```python
from build123d import *

# Parameters (mm, degrees)
SKETCH1_R               = 6.477
BOSS_EXTRUDE1_DEPTH     = 2.032
CUT_EXTRUDE1_DEPTH      = 0.64008
SKETCH3_W               = 1.19888
SKETCH3_H               = 8.98144
CUT_EXTRUDE2_DEPTH      = 1.09982
SKETCH4_W               = 7.19836
SKETCH4_H               = 7.00786
CUT_EXTRUDE3_DEPTH      = 0.8001
BOSS_EXTRUDE2_DEPTH     = 1.27
SKETCH6_W               = 2.286
SKETCH6_H               = 1.99898
BOSS_EXTRUDE3_DEPTH     = 2.54
SKETCH7_R               = 3.3734375
BOSS_EXTRUDE4_DEPTH     = 2.032
SKETCH8_W               = 2.54
SKETCH8_H               = 0.79375
CUT_EXTRUDE4_DEPTH      = 1
CUT_EXTRUDE4_DEPTH_BACK = 29.6004
CHAMFER1_SIZE           = 1.143
CHAMFER2_SIZE           = 1.143


with BuildPart() as part:
    # Sketch1 → Boss-Extrude1 (new body)
    with BuildSketch(Plane(origin=(0, 0, 0), x_dir=(1, 0, 0), z_dir=(0, 1, 0))):
        with BuildLine():
            Line((-14.3002, 5.9944), (-14.3002, -24.3332))
            Line((-14.3002, -24.3332), (-9.271, -28.0416))
            Line((-9.271, -28.0416), (9.271, -28.0416))
            Line((9.271, -28.0416), (14.3002, -24.3332))
            Line((14.3002, -24.3332), (14.3002, 5.9944))
            ThreePointArc((14.3002, 5.9944), (0, 15.505758653), (-14.3002, 5.9944))
        make_face()
        Circle(SKETCH1_R, mode=Mode.SUBTRACT)
    extrude(amount=BOSS_EXTRUDE1_DEPTH)

    # Sketch2 → Cut-Extrude1 (cut)
    with BuildSketch(Plane(origin=(0, 2.032, 0), x_dir=(1, 0, 0), z_dir=(0, 1, 0))):
        Polygon((0, -28.0416), (-7.71906, -28.0416), (-7.71906, -16.06042), (7.71906, -16.06042), (7.71906, -28.0416), align=None)
    extrude(amount=-CUT_EXTRUDE1_DEPTH, mode=Mode.SUBTRACT)

    # Sketch3 → Cut-Extrude2 (cut)
    with BuildSketch(Plane(origin=(0, 1.39192, 0), x_dir=(1, 0, 0), z_dir=(0, 1, 0))):
        with Locations((-5.06984, -23.55088)):
            Rectangle(SKETCH3_W, SKETCH3_H)
        with Locations((2.52984, -23.55088)):
            Rectangle(SKETCH3_W, SKETCH3_H)
    extrude(amount=-CUT_EXTRUDE2_DEPTH, mode=Mode.SUBTRACT)

    # Sketch4 → Cut-Extrude3 (cut)
    with BuildSketch(Plane(origin=(0, 2.032, 0), x_dir=(1, 0, 0), z_dir=(0, 1, 0))):
        with Locations((-3.299968, -11.116564)):
            Rectangle(SKETCH4_W, SKETCH4_H)
    extrude(amount=-CUT_EXTRUDE3_DEPTH, mode=Mode.SUBTRACT)

    # Sketch5 → Boss-Extrude2 (add)
    with BuildSketch(Plane(origin=(0, 2.032, 0), x_dir=(1, 0, 0), z_dir=(0, 1, 0))):
        with BuildLine():
            Line((12.40282, -22.33422), (13.171678, -22.33422))
            Line((13.171678, -22.33422), (13.40104, -22.152864))
            Line((13.40104, -22.152864), (13.40104, 4.882896))
            ThreePointArc((13.40104, 4.882896), (13.360125716, 5.283490726), (13.23975, 5.667756))
            ThreePointArc((13.23975, 5.667756), (10.160746855, 10.20631074), (5.608066, 13.264388))
            ThreePointArc((5.608066, 13.264388), (5.250053957, 13.366581837), (4.87934, 13.40104))
            Line((4.87934, 13.40104), (4.50342, 13.40104))
            Line((4.50342, 13.40104), (4.50342, 12.40282))
            Line((4.50342, 12.40282), (4.87934, 12.40282))
            ThreePointArc((4.87934, 12.40282), (5.080028543, 12.382451063), (5.272532, 12.322175))
            ThreePointArc((5.272532, 12.322175), (9.477779109, 9.479294357), (12.322175, 5.275072))
            ThreePointArc((12.322175, 5.275072), (12.382451063, 5.082568543), (12.40282, 4.88188))
            Line((12.40282, 4.88188), (12.40282, -22.33422))
        make_face()
        with BuildLine():
            Line((-4.850750436, 13.40104), (-4.474830436, 13.40104))
            Line((-4.474830436, 13.40104), (-4.474830436, 12.40282))
            Line((-4.474830436, 12.40282), (-4.850750436, 12.40282))
            ThreePointArc((-4.850750436, 12.40282), (-5.051438979, 12.382451063), (-5.243942436, 12.322175))
            ThreePointArc((-5.243942436, 12.322175), (-9.449189546, 9.479294357), (-12.293585436, 5.275072))
            ThreePointArc((-12.293585436, 5.275072), (-12.353861499, 5.082568543), (-12.374230436, 4.88188))
            Line((-12.374230436, 4.88188), (-12.374230436, -22.33422))
            Line((-12.374230436, -22.33422), (-13.143088436, -22.33422))
            Line((-13.143088436, -22.33422), (-13.372450436, -22.152864))
            Line((-13.372450436, -22.152864), (-13.372450436, 4.882896))
            ThreePointArc((-13.372450436, 4.882896), (-13.331536152, 5.283490726), (-13.211160436, 5.667756))
            ThreePointArc((-13.211160436, 5.667756), (-10.132157291, 10.20631074), (-5.579476436, 13.264388))
            ThreePointArc((-5.579476436, 13.264388), (-5.221464393, 13.366581837), (-4.850750436, 13.40104))
        make_face()
    extrude(amount=BOSS_EXTRUDE2_DEPTH)

    # Sketch6 → Boss-Extrude3 (add)
    with BuildSketch(Plane(origin=(0, 1.39192, 0), x_dir=(1, 0, 0), z_dir=(0, 1, 0))):
        with Locations((6.57606, -27.04211)):
            Rectangle(SKETCH6_W, SKETCH6_H)
    extrude(amount=BOSS_EXTRUDE3_DEPTH)

    # Sketch7 → Boss-Extrude4 (add)
    with BuildSketch(Plane.XZ):
        with BuildLine():
            Line((-6.35, -25.4), (-6.35, -22.86))
            ThreePointArc((-6.35, -22.86), (-7.612456929, -16.312404928), (-11.218821547, -10.703578583))
            ThreePointArc((-11.218821547, -10.703578583), (0, -15.505758653), (11.218821547, -10.703578583))
            ThreePointArc((11.218821547, -10.703578583), (7.612456929, -16.312404928), (6.35, -22.86))
            Line((6.35, -22.86), (6.35, -25.4))
            ThreePointArc((6.35, -25.4), (0, -31.75), (-6.35, -25.4))
        make_face()
        with Locations((0, -25.4)):
            Circle(SKETCH7_R, mode=Mode.SUBTRACT)
    extrude(amount=-BOSS_EXTRUDE4_DEPTH)

    # Sketch8 → Cut-Extrude4 (cut, two sides)
    with BuildSketch(Plane(origin=(14.3002, 0, 0), x_dir=(0, 0, -1), z_dir=(1, 0, 0))) as cut_extrude4_sk:
        with Locations((-11.43, 0.396875)):
            Rectangle(SKETCH8_W, SKETCH8_H)
    extrude(amount=CUT_EXTRUDE4_DEPTH, mode=Mode.SUBTRACT)
    extrude(cut_extrude4_sk.sketch, amount=-CUT_EXTRUDE4_DEPTH_BACK, mode=Mode.SUBTRACT)

    # Chamfer1
    chamfer1_edges = [part.edges().sort_by_distance(p)[0] for p in [
        (14.3002, 0.79375, 11.43),
    ]]
    chamfer(chamfer1_edges, length=CHAMFER1_SIZE)

    # Chamfer2
    chamfer2_edges = [part.edges().sort_by_distance(p)[0] for p in [
        (-14.3002, 0.79375, 11.43),
    ]]
    chamfer(chamfer2_edges, length=CHAMFER2_SIZE)


solid = part.part
```
Build history of the part. All positions in model axes, mm. A direction names the side the tool comes from. Give positions to 0.01 mm unless a question says otherwise; leave off trailing zeros. Loops run counter-clockwise (first coordinate to the right, second up) from the corner with the lowest first, then second, coordinate; pieces in that order, holes last. Notation, with made-up numbers: (78.25, 8) -> (124.25, 8) arc R14 ccw to (124.25, 12) -> close; hole circle Ø11 at (59.5, -38.75). An arc over 180 degrees is marked (long way). One line per question, with ' | ' between items.
Q1. Pull direction X, two halves, no side cores. Call faces 4 (the flat face through (7, 3.932, 27)), 5 (the flat face through (4.503, 3, -13)), 6 (the flat face through (3.129, 1, 24)), 7 (the flat face through (13.721, 1.357, 11.448)): pulls with the +X half, pulls with the -X half, needs draft (parallel to the pull), parting line crosses it, or undercut.
Filled sheet:
face 4: needs draft | face 5: undercut | face 6: undercut | face 7: pulls with the +X half
Q2. Cut at A-A, the plane y = 2.6. Count the separate pieces of the cut face and the enclosed holes in it, plus the area to 3 significant figures.
Filled sheet:
separate pieces: 3 | enclosed holes: 0 | area: 83.2 mm²
Q3. Drop flat-ended pins along their axis: pin 1 (1.6 mm diameter, centred on y = 0.5, z = -24.5, fed in from +X); pin 2 (0.9 mm diameter, centred on y = 3.5, z = 27, fed in from +X); pin 3 (0.8 mm diameter, centred on y = 2.5, z = -13, fed in from +X). Give the stop position or say it passes through.
Filled sheet:
pin 1: stops at x = 6.35 | pin 2: stops at x = 7.72 | pin 3: stops at x = 6.97
Q4. Cut at B-B, the plane z = 5.5. Write the cut outline in (x, y), plus the area to 3 significant figures.
Filled sheet:
outline: (-14.3, 0) -> (-3.42, 0) -> (-3.42, 2.03) -> (-12.37, 2.03) -> (-12.37, 3.3) -> (-13.37, 3.3) -> (-13.37, 2.03) -> (-14.3, 2.03) -> close; (3.42, 0) -> (14.3, 0) -> (14.3, 2.03) -> (13.4, 2.03) -> (13.4, 3.3) -> (12.4, 3.3) -> (12.4, 2.03) -> (3.42, 2.03) -> close | area: 46.7 mm²
Q5. Tool access for faces 1 (the flat face through (2.5, 0.292, 23.5)), 2 (the cylindrical face through (10.215, 2.658, -10.152)), 3 (the flat face through (6.35, 1, -24)): list every direction of +Z, -Z, +X, -X, +Y, -Y with a clear straight run to the whole face (end or side of a thin tool).
Filled sheet:
face 1: +Z, +Y | face 2: -Z, +X, +Y | face 3: -Z, +X, +Y, -Y
Q6. Cut at D-D, the plane z = -18.5. Write the cut outline in (x, y).
Filled sheet:
outline: (-6.9, 0) -> (6.9, 0) -> (6.9, 2.03) -> (-6.9, 2.03) -> close
Q7. Drill centre lines: line 1 along Z through (x, y) = (0, 1); line 2 along Z through (x, y) = (0, 0.75); line 3 along X through (y, z) = (0.9, 24). Where is each one in solid material? Low to high. Write a range as [from, to].
Filled sheet:
line 1: z = [-31.75, -28.77], [-22.03, -6.48], [6.48, 28.04] | line 2: z = [-31.75, -28.77], [-22.03, -6.48], [6.48, 10.16], [12.7, 28.04] | line 3: x = [-14.3, -5.67], [-4.47, 1.93], [3.13, 14.3]
Q8. Cut at C-C, the plane x = -0.5. Write the cut outline in (y, z).
Filled sheet:
outline: (0, -31.73) -> (2.03, -31.73) -> (2.03, -28.74) -> (0, -28.74) -> close; (0, -22.06) -> (2.03, -22.06) -> (2.03, -6.46) -> (0, -6.46) -> close; (0, 6.46) -> (2.03, 6.46) -> (2.03, 7.61) -> (1.23, 7.61) -> (1.23, 14.62) -> (2.03, 14.62) -> (2.03, 16.06) -> (1.39, 16.06) -> (1.39, 28.04) -> (0, 28.04) -> (0, 12.7) -> (0.79, 12.7) -> (0.79, 10.16) -> (0, 10.16) -> close
